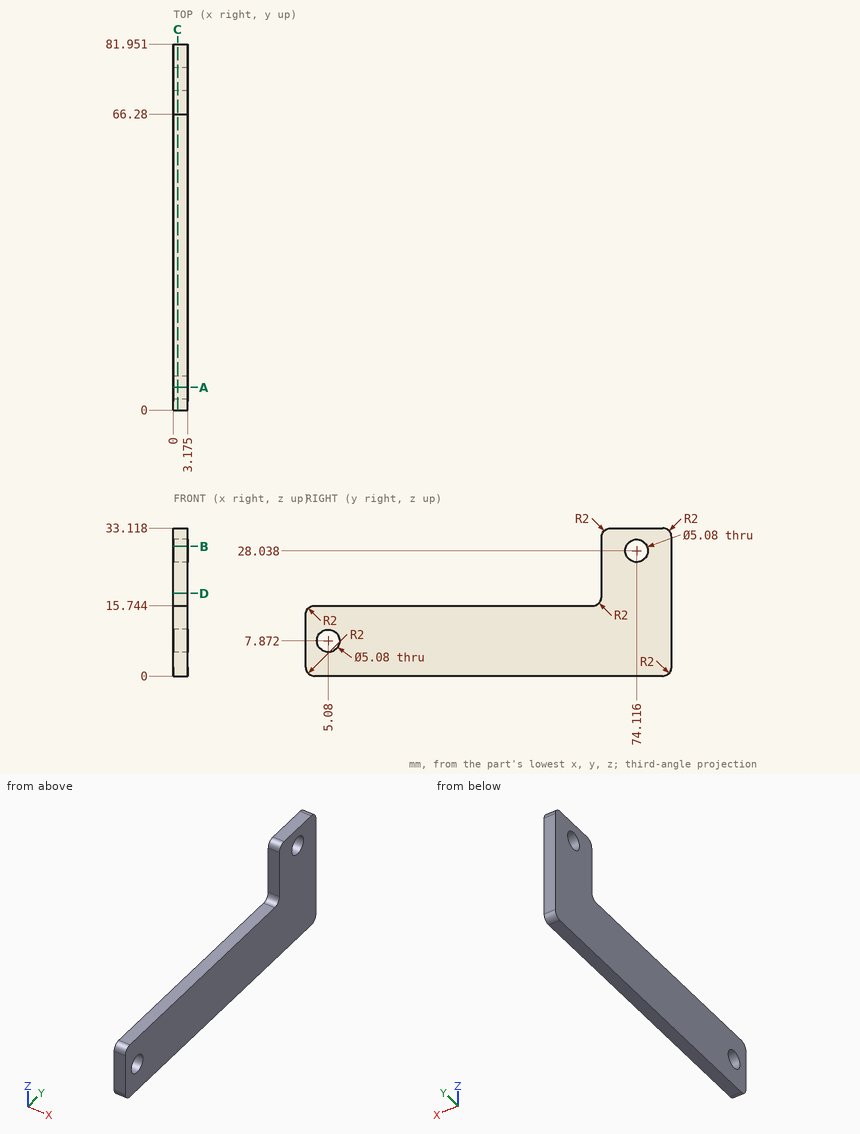
Geometry: see drawing. Coordinates: mm, zero at the bounding-box minimum. Give positions to 0.01 mm unless a question says otherwise; leave off trailing zeros. Write each loop counter-clockwise with the first axis right and the second up, starting at its lowest first coordinate (ties: lowest second). Pieces come first, ordered by that corner, then holes. Notation, with made-up numbers: (70.5, 62.5) -> (110.5, 62.5) arc R20 cw to (110.5, 97.5) -> close; hole circle Ø7 at (-31.75, 41.25). An arc over 180 degrees is marked (long way). Use one line per item in the form item = value. Start each with the question number.
1) Section query C-C on x = 0.95. Return the cut outline in (y, z) (1 decimal).
2) Section query A-A on y = 5.08. Return the cut outline in (x, z) (1 decimal).
3) Section query B-B on z = 29. Return the cut outline in (x, y) (1 decimal).
4) Ray query, probe 1 along Z at (x, y) = (2.45, 55.5); probe 2 along Y at (x, z) = (2.75, 24); probe 3 along Z at (x, y) = (2.65, 72) (1 decimal). Return the intervals inside material, ascending. Write a range as from..to.
5) Section query D-D on z = 18.5. Return the cut outline in (x, y) (1 decimal).
6) Pin query (flat end, axial travel): pin 1 (1 mm diameter, centred on x = 1.5, z = 22.5, fed in from -Y). Return the tip coordinate at first contact, or that it passes through.
Outcome:
q1.outline = (0, 2) arc R2 ccw to (2, 0) -> (80, 0) arc R2 ccw to (82, 2) -> (82, 31.1) arc R2 ccw to (80, 33.1) -> (68.3, 33.1) arc R2 ccw to (66.3, 31.1) -> (66.3, 17.7) arc R2 cw to (64.3, 15.7) -> (2, 15.7) arc R2 ccw to (0, 13.7) -> close; hole circle Ø5.1 at (5.1, 7.9); hole circle Ø5.1 at (74.1, 28)
q2.outline = (0, 0) -> (3.2, 0) -> (3.2, 5.3) -> (0, 5.3) -> close; (0, 10.4) -> (3.2, 10.4) -> (3.2, 15.7) -> (0, 15.7) -> close
q3.outline = (0, 66.3) -> (3.2, 66.3) -> (3.2, 71.8) -> (0, 71.8) -> close; (0, 76.5) -> (3.2, 76.5) -> (3.2, 82) -> (0, 82) -> close
q4.probe_1 = 0..15.74
q4.probe_2 = 66.28..81.95
q4.probe_3 = 0..26.6, 29.4..33.1
q5.outline = (0, 66.3) -> (3.2, 66.3) -> (3.2, 82) -> (0, 82) -> close
q6.pin_1 = 66.28
